Could you check a few things on this model? Use its own coordinates, in mm. Coordinates: 2 decimals unless noted, no trailing zeros. Write each loop counter-clockwise with the first axis right and the second up, starting at its lowest first coordinate (ties: lowest second). Pieces come first, ordered by that corner, then holes. Notation, with made-up numbers: M -15,4 L -10,4 A29 ccw -10,27 Z; hole C 83,83 d11. An arc over 180 degrees is marked long. Write item = value, one per line.
```python
from build123d import *

# Parameters (mm, degrees)
SKETCH_1_R      = 5.1
SKETCH_1_R_2    = 1.7
SKETCH_1_R_3    = 2
SKETCH_1_R_4    = 7.5
SKETCH_1_R_5    = 6
SKETCH_1_R_6    = 2.5
EXTRUDE_1_DEPTH = 6


with BuildPart() as part:
    # 草图1 → 凸台-拉伸1 (new body)
    with BuildSketch(Plane(origin=(0, 0, 0), x_dir=(1, 0, 0), z_dir=(0, 1, 0))):
        Polygon((0, 200), (25, 200), (25, 206), (75, 206), (75, 200), (125, 200), (125, 206), (175, 206), (175, 200), (200, 200), (200, 175), (206, 175), (206, 125), (200, 125), (200, 75), (206, 75), (206, 25), (200, 25), (200, 0), (175, 0), (175, -6), (125, -6), (125, 0), (75, 0), (75, -6), (25, -6), (25, 0), (0, 0), (0, 25), (-6, 25), (-6, 75), (0, 75), (0, 125), (-6, 125), (-6, 175), (0, 175), align=None)
        with Locations(Location((100, 100, 0), (0, 0, 270))):
            Circle(SKETCH_1_R, mode=Mode.SUBTRACT)
        with Locations(Location((150, 112, 0), (0, 0, 270))):
            Circle(SKETCH_1_R_2, mode=Mode.SUBTRACT)
        with Locations(Location((100, 108, 0), (0, 0, 270))):
            Circle(SKETCH_1_R_3, mode=Mode.SUBTRACT)
        with Locations(Location((108, 100, 0), (0, 0, 270))):
            Circle(SKETCH_1_R_3, mode=Mode.SUBTRACT)
        with Locations(Location((100, 92, 0), (0, 0, 270))):
            Circle(SKETCH_1_R_3, mode=Mode.SUBTRACT)
        with Locations(Location((92, 100, 0), (0, 0, 270))):
            Circle(SKETCH_1_R_3, mode=Mode.SUBTRACT)
        with Locations(Location((50, 100, 0), (0, 0, 270))):
            Circle(SKETCH_1_R_4, mode=Mode.SUBTRACT)
        with Locations(Location((50, 112, 0), (0, 0, 270))):
            Circle(SKETCH_1_R_2, mode=Mode.SUBTRACT)
        with Locations(Location((62, 100, 0), (0, 0, 270))):
            Circle(SKETCH_1_R_2, mode=Mode.SUBTRACT)
        with Locations(Location((50, 88, 0), (0, 0, 270))):
            Circle(SKETCH_1_R_2, mode=Mode.SUBTRACT)
        with Locations(Location((38, 100, 0), (0, 0, 270))):
            Circle(SKETCH_1_R_2, mode=Mode.SUBTRACT)
        with Locations(Location((162, 100, 0), (0, 0, 270))):
            Circle(SKETCH_1_R_2, mode=Mode.SUBTRACT)
        with Locations(Location((138, 100, 0), (0, 0, 270))):
            Circle(SKETCH_1_R_2, mode=Mode.SUBTRACT)
        with Locations(Location((150, 88, 0), (0, 0, 270))):
            Circle(SKETCH_1_R_2, mode=Mode.SUBTRACT)
        with Locations(Location((150, 100, 0), (0, 0, 270))):
            Circle(SKETCH_1_R_4, mode=Mode.SUBTRACT)
        with Locations(Location((100, 160, 0), (0, 0, 270))):
            Circle(SKETCH_1_R_5, mode=Mode.SUBTRACT)
        with Locations(Location((-3, 150, 0), (0, 0, 270))):
            Circle(SKETCH_1_R_6, mode=Mode.SUBTRACT)
        with Locations(Location((203, 150, 0), (0, 0, 270))):
            Circle(SKETCH_1_R_6, mode=Mode.SUBTRACT)
        with Locations(Location((203, 50, 0), (0, 0, 270))):
            Circle(SKETCH_1_R_6, mode=Mode.SUBTRACT)
        with Locations(Location((-3, 50, 0), (0, 0, 270))):
            Circle(SKETCH_1_R_6, mode=Mode.SUBTRACT)
    extrude(amount=EXTRUDE_1_DEPTH)


solid = part.part
```
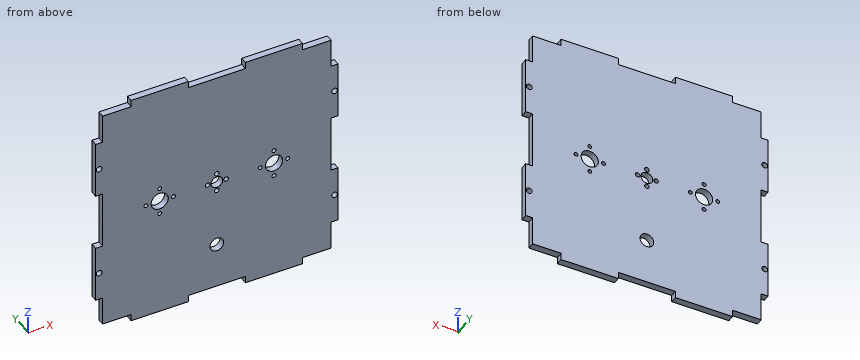
Item 1: Imagine slicing it at D-D (x = 19.5). Write out the boundary of the cut face in (y, z).
Numbers:
outline = M 0,-200 L 6,-200 L 6,0 L 0,0 Z
Item 2: I'm going to push flat-ended pins straight in: P1, Ø1.8, axis at y = 4, z = -188, coming from the +X side; P2, Ø3, axis at y = 3, z = -90.5, coming from the -X side. Where does each tip first touch, or does it pass through?
Numbers:
P1 = 200
P2 = 0
Item 3: Imagine slicing it at A-A (z = -160). Write out the boundary of the cut face in (x, y), and give its area (3 significant figures).
Numbers:
outline = M -6,0 L 94,0 L 94,6 L -6,6 Z; M 106,0 L 206,0 L 206,6 L 106,6 Z
area = 1,200 mm²
Item 4: Imagine slicing it at C-C (z = -184). Write out the boundary of the cut face in (x, y).
Numbers:
outline = M 0,0 L 200,0 L 200,6 L 0,6 Z
Item 5: Imagine slicing it at B-B (y = 4.45). State how many separate pieces and enclosed holes the cut face has, and give its area (3 significant figures).
Numbers:
separate_pieces = 1
enclosed_holes = 20
area = 41,700 mm²
Item 6: If I drill on line 1 along Z through (x, y) = (203, 3.95); line 2 along Z through (x, y) = (45.5, 2.5); line 3 along X through (y, z) = (3.5, -50), over which ranges is the centre line in solid material (lowest first)?
Numbers:
line_1 = -175 to -152.5, -147.5 to -125, -75 to -52.5, -47.5 to -25
line_2 = -206 to -106, -94 to 6
line_3 = -6 to -5.5, -0.5 to 200.5, 205.5 to 206
